Autodesk Inventor part; units mm, degrees
ref_plane "YZ Plane" through (0, 0, 0) normal (1, 0, 0) x (0, 1, 0)
ref_plane "XZ Plane" through (0, 0, 0) normal (0, 1, 0) x (-1, 0, 0)
ref_plane "XY Plane" through (0, 0, 0) normal (0, 0, 1) x (1, 0, 0)
sketch "Sketch1" plane through (0, 0, 0) normal (1, 0, 0) x (0, 1, 0)
  line L0 (0, 0) -> (50.8, 0)
  line L1 (50.8, 0) -> (50.8, -25.4)
  line L2 (50.8, -25.4) -> (0, -25.4)
  line L3 (0, -25.4) -> (0, 0)
  line L4 (47.625, -3.175) -> (3.175, -3.175)
  line L5 (3.175, -3.175) -> (3.175, -22.225)
  line L6 (3.175, -22.225) -> (47.625, -22.225)
  line L7 (47.625, -22.225) -> (47.625, -3.175)
  dimension "d0" = 50.8
  dimension "d1" = 25.4
  dimension "d2" = 3.175
extrude "Extrusion1" add sketch "Sketch1" along normal blind 101.6
sketch "Sketch2" plane through (0, 0, -25.4) normal (0, 0, -1) x (-1, 0, 0)
  line L0 (0, 50.8) -> (-101.6, 50.8)
  line L1 (0, 50.8) -> (0, 0)
  line L2 (0, 0) -> (-101.6, 0)
  point P0 (-25.4, 25.4)
  dimension "d5" = 25.4
  dimension "d6" = 25.4
hole "Hole1" at (25.4, 25.4, -25.4) direction (0, 0, 1) diameter 28.575 depth 3.175 tip angle 118
hole "Hole2" at (25.4, 25.4, -25.4) direction (0, 0, 1) diameter 15.875 end through all
properties part number "15102898-16-P-0304" material "Aluminum 6061"
Geometry: final body of the model. Coordinates: model frame, mm. A direction names the side the tool comes from. Round coordinates to 2 decimals unless told otherwise and drop trailing zeros. Loops run counter-clockwise (first coordinate to the right, second up) from the corner with the lowest first, then second, coordinate; pieces in that order, holes last.
Item 1: Line query: L1, parallel to Y at x = 81.5, z = -8.75 (3 decimals); L2, parallel to Z at x = 47, y = 23 (3 decimals); L3, parallel to Y at x = 25.4, z = -24.5. Output: solid intervals per line, ascending.
Checked values:
L1: y = 0 to 3.175, 47.625 to 50.8
L2: z = -25.4 to -22.225, -3.175 to 0
L3: y = 0 to 11.11, 39.69 to 50.8
Item 2: Mould query, pull axis Z, two halves, no side actions, for faces 4 (the flat face through (50, 25, -22.225)), 5 (the flat face through (50, 0, -13)), 6 (the flat face through (50, 26, -3.175)), 7 (the flat face through (50, 26, -25.4)). Classes: released by +Z, released by -Z, zero draft, split by the parting line, or undercut.
Checked values:
face 4: undercut
face 5: zero draft
face 6: undercut
face 7: released by -Z
Item 3: Section D-D, the plane y = 9.5. Output: boundary loops of the cut face in (x, z) (3 decimals), plus the area to 3 significant figures.
Checked values:
outline: (0, -25.4) - (101.6, -25.4) - (101.6, -22.225) - (0, -22.225) - close; (0, -3.175) - (101.6, -3.175) - (101.6, 0) - (0, 0) - close
area: 645 mm2
Item 4: Reachability of faces 1 (the flat face through (50, 47.625, -13)), 2 (the cylindrical face through (15.744, 14.87, -23.79)), 3 (the flat face through (50, 25, 0)) from +Z, -Z, +X, -X, +Y, -Y: full face, straight path, thin tool, end or side. Return the list, or none.
Checked values:
face 1: +X, -X
face 2: -Z
face 3: +Z, +X, -X, +Y, -Y
Item 5: Section B-B, the plane x = 25.4. Output: boundary loops of the cut face in (y, z) (1 decimal).
Checked values:
outline: (0, -25.4) - (11.1, -25.4) - (11.1, -22.2) - (3.2, -22.2) - (3.2, -3.2) - (17.5, -3.2) - (17.5, 0) - (0, 0) - close; (33.3, -3.2) - (47.6, -3.2) - (47.6, -22.2) - (39.7, -22.2) - (39.7, -25.4) - (50.8, -25.4) - (50.8, 0) - (33.3, 0) - close
Item 6: Contact query for flat-ended pins moving along their axis: P1, Ø10, axis at x = 18.5, z = -11, coming from the -Y side; P2, Ø17, axis at x = 25.4, y = 25.4, coming from the -Z side (3 decimals). Output: stop coordinate, or through.
Checked values:
P1: stops at y = 0
P2: stops at z = -3.175
Item 7: Section A-A, the plane y = 25.4. Output: boundary loops of the cut face in (x, z) (1 decimal), plus the area to 3 significant figures.
Checked values:
outline: (0, -25.4) - (11.1, -25.4) - (11.1, -22.2) - (0, -22.2) - close; (0, -3.2) - (17.5, -3.2) - (17.5, 0) - (0, 0) - close; (33.3, -3.2) - (101.6, -3.2) - (101.6, 0) - (33.3, 0) - close; (39.7, -25.4) - (101.6, -25.4) - (101.6, -22.2) - (39.7, -22.2) - close
area: 504 mm2
Item 8: Section C-C, the plane z = -4.75. Output: boundary loops of the cut face in (x, y) (3 decimals), plus the area to 3 significant figures.
Checked values:
outline: (0, 0) - (101.6, 0) - (101.6, 3.175) - (0, 3.175) - close; (0, 47.625) - (101.6, 47.625) - (101.6, 50.8) - (0, 50.8) - close
area: 645 mm2
